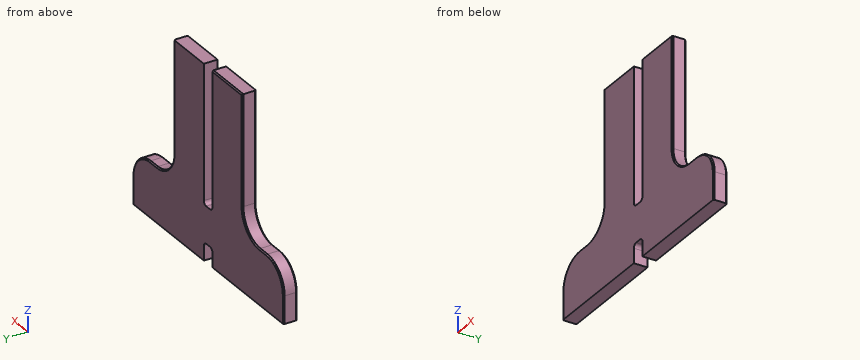
from build123d import *

# Parameters (mm, degrees)
F1_DEPTH = 19.05
F2_R     = 38.1
F3_R     = 5.08
F4_SIZE  = 1.5875


with BuildPart() as f1:
    # F0 (on Front) → F1 (new body)
    with BuildSketch(Plane.XZ):
        Polygon((76.2, -95.25), (76.2, 95.25), (9.525, 95.25), (9.525, -95.25), (-9.525, -95.25), (-9.525, 95.25), (-76.2, 95.25), (-76.2, -95.25), (-168.275, -95.25), (-168.275, -171.45), (-9.525, -171.45), (-9.525, -146.05), (9.525, -146.05), (9.525, -171.45), (168.275, -171.45), (168.275, -95.25), align=None)
    extrude(amount=F1_DEPTH)

    # F2
    f2_edges = [f1.edges().sort_by_distance(p)[0] for p in [
        (-168.275, -9.525, -95.25),
        (-76.2, -9.525, -95.25),
        (76.2, -9.525, -95.25),
        (168.275, -9.525, -95.25),
    ]]
    fillet(f2_edges, radius=F2_R)

    # F3
    f3_edges = [f1.edges().sort_by_distance(p)[0] for p in [
        (9.525, -9.525, -95.25),
        (-9.525, -9.525, -95.25),
        (-9.525, -9.525, -146.05),
        (9.525, -9.525, -146.05),
    ]]
    fillet(f3_edges, radius=F3_R)

    # F4
    f4_edges = [f1.edges().sort_by_distance(p)[0] for p in [
        (-122.2375, -19.05, -95.25),
        (122.2375, -19.05, -95.25),
        (122.2375, 0, -95.25),
        (-42.8625, 0, 95.25),
        (-76.2, 0, 19.05),
        (-122.2375, 0, -95.25),
    ]]
    chamfer(f4_edges, length=F4_SIZE)


solid = f1.part
Read the model definition and answer for the solid it produces. Units are mm, in the model's axes. Give positions to 0.01 mm unless a question says otherwise; leave off trailing zeros. Loops run counter-clockwise (first coordinate to the right, second up) from the corner with the lowest first, then second, coordinate; pieces in that order, holes last. Notation, with made-up numbers: (25, 39.5) -> (78, 39.5) arc R22 cw to (78, 74.5) -> close; hole circle Ø9 at (23, -29.75). An arc over 180 degrees is marked (long way). Use a Markdown table: item, result.
Q1. Find the intervals of material crossed by line 1 along X through (y, z) = (-17.5, -21.5) (1 decimal); line 2 along X through (y, z) = (-12.25, -156) (3 decimals); line 3 along Z through (x, y) = (-131, -3.5), in increasing order.
Solved:
| item | result |
|---|---|
| line 1 | x = -76.2 to -9.5, 9.5 to 76.2 |
| line 2 | x = -168.275 to -9.525, 9.525 to 168.275 |
| line 3 | z = -171.45 to -95.26 |
Q2. Section B-B, the plane x = -118.5 is taken. Determine the outline of the cut face in (y, z).
Solved:
| item | result |
|---|---|
| outline | (-19.05, -171.45) -> (0, -171.45) -> (0, -96.84) -> (-1.59, -95.25) -> (-17.46, -95.25) -> (-19.05, -96.84) -> close |
Q3. Section C-C, the plane y = -13.5 is taken. Determine the outline of the cut face in (x, z) (3 decimals), then the cut area to 3 significant figures.
Solved:
| item | result |
|---|---|
| outline | (-168.275, -171.45) -> (-9.525, -171.45) -> (-9.525, -151.13) arc R5.08 cw to (-4.445, -146.05) -> (4.445, -146.05) arc R5.08 cw to (9.525, -151.13) -> (9.525, -171.45) -> (168.275, -171.45) -> (168.275, -133.35) arc R38.1 ccw to (130.175, -95.25) -> (114.3, -95.25) arc R38.1 cw to (76.2, -57.15) -> (76.2, 95.25) -> (9.525, 95.25) -> (9.525, -90.17) arc R5.08 cw to (4.445, -95.25) -> (-4.445, -95.25) arc R5.08 cw to (-9.525, -90.17) -> (-9.525, 95.25) -> (-76.2, 95.25) -> (-76.2, -57.15) arc R38.1 cw to (-114.3, -95.25) -> (-130.175, -95.25) arc R38.1 ccw to (-168.275, -133.35) -> close |
| area | 50,600 mm^2 |
Q4. Each of these flat-tipped pins is pushed along its axis until it touches: pin 1 (5 mm diameter, centred on y = -7.5, z = 50.5, fed in from -X); pin 2 (5 mm diameter, centred on x = 102.5, y = -4, fed in from +Z); pin 3 (7 mm diameter, centred on x = -1.5, y = -12.5, fed in from +Z). Where does it stop, or does it pass through?
Solved:
| item | result |
|---|---|
| pin 1 | stops at x = -76.2 |
| pin 2 | stops at z = -92.46 |
| pin 3 | stops at z = -95.22 |
